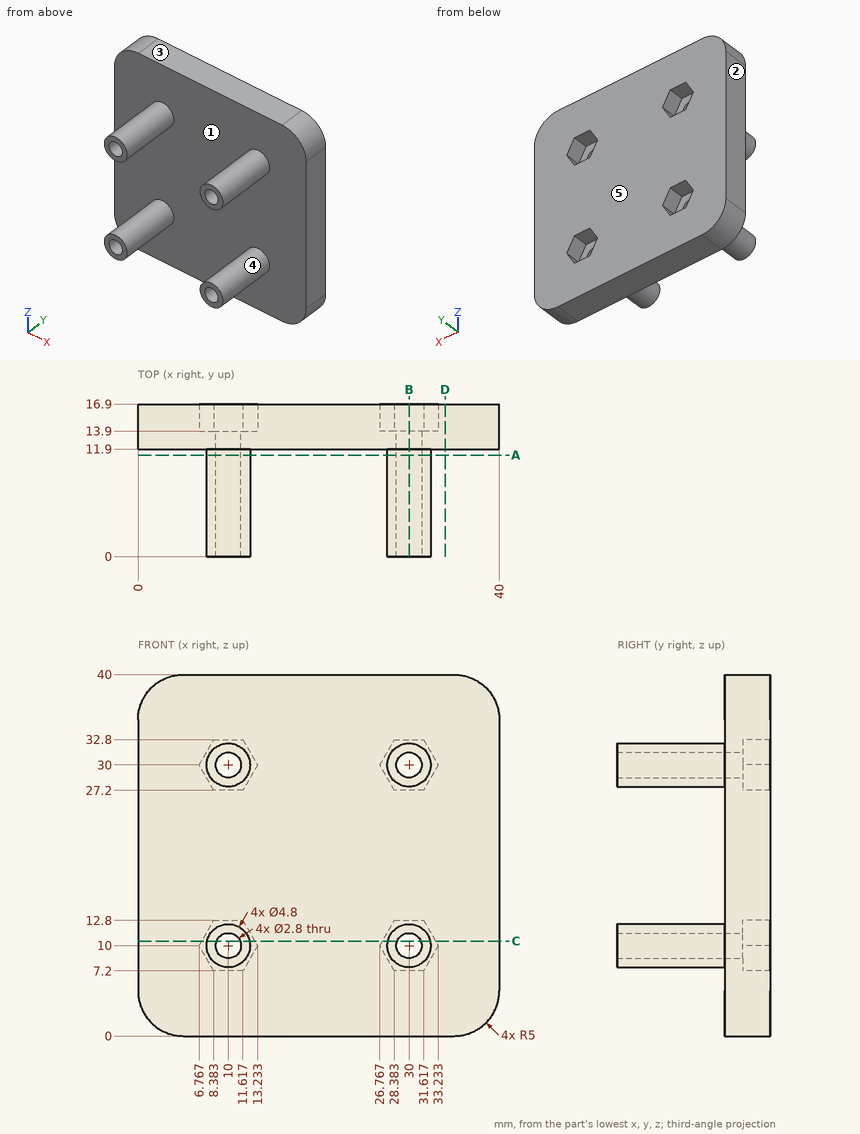
Design review of the part shown in the three views and the two pictorial views. Dimensions are in mm from the part's minimum x, y and z. A direction names the side the tool comes from. Give positions to 0.01 mm unless a question says otherwise; leave off trailing zeros. Order: outer loops, then holes, each group sorted by start corner. A loop starts at its lowest first (then second) coordinate and runs counter-clockwise, first axis right, second up. Notation, with made-up numbers: M -0.5,71 L 9.5,71 A26 cw 9.5,106 Z; hole C 69,1 d1. An arc over 180 degrees is marked long. Answer in a Markdown table with one row per item. Add a question column.
(1) Consider section D-D on x = 34. State the section outline as (y, z) points.
(2) For the marked faces 1 and 2, list the 3-axis set-ups (+Z, -Z, +X, -X, +Y, -Y) from which the entire face can be reached by the end or side of a thin tool; tool diameter is ignored.
(3) Consider section C-C on z = 10.5. State the section outline as (x, y) points (1 decimal).
(4) For pin 1 (3 mm diameter, centred on x = 9.5, z = 11, fed in from +Y); pin 2 (6 mm diameter, centred on y = 5, z = 29, fed in from -X), all flat-tipped, find the tip position at first contact; note any pin that passes through.
(5) Wall thickness on probe 1 along X at (y, z) = (10.5, 10); probe 2 along Z at (x, y) = (31, 12.25): over which ranges is each line inside the solid? List them lowest first. Write a range as [from, to].
(6) Consider section B-B on x = 30. State the section outline as (y, z) points, and give its area (3 significant figures).
(7) Mouldability with a two-part tool opening along Z and no side actions: class the marked faces 3, 4 and 5 as +Z half, -Z half, draft (parallel to the pull), parting line (faces both ways), or undercut.
(8) Consider section A-A on y = 11.25. State the section outline as (x, z) points.
Evaluation:
| question | item | result |
|---|---|---|
| 1 | outline | M 11.9,0 L 16.9,0 L 16.9,40 L 11.9,40 Z |
| 2 | face 1 | -Y |
| 2 | face 2 | +Z, -Z, -X, +Y, -Y |
| 3 | outline | M 0,11.9 L 7.7,11.9 L 7.7,0 L 8.7,0 L 8.7,13.9 L 7.1,13.9 L 7.1,16.9 L 0,16.9 Z; M 11.3,0 L 12.3,0 L 12.3,11.9 L 27.7,11.9 L 27.7,0 L 28.7,0 L 28.7,13.9 L 27.1,13.9 L 27.1,16.9 L 12.9,16.9 L 12.9,13.9 L 11.3,13.9 Z; M 31.3,0 L 32.3,0 L 32.3,11.9 L 40,11.9 L 40,16.9 L 32.9,16.9 L 32.9,13.9 L 31.3,13.9 Z |
| 4 | pin 1 | stops at y = 13.9 |
| 4 | pin 2 | stops at x = 7.6 |
| 5 | probe 1 | x = [7.6, 8.6], [11.4, 12.4], [27.6, 28.6], [31.4, 32.4] |
| 5 | probe 2 | z = [0, 9.02], [10.98, 29.02], [30.98, 40] |
| 6 | outline | M 0,7.6 L 11.9,7.6 L 11.9,0 L 16.9,0 L 16.9,7.2 L 13.9,7.2 L 13.9,8.6 L 0,8.6 Z; M 0,11.4 L 13.9,11.4 L 13.9,12.8 L 16.9,12.8 L 16.9,27.2 L 13.9,27.2 L 13.9,28.6 L 0,28.6 L 0,27.6 L 11.9,27.6 L 11.9,12.4 L 0,12.4 Z; M 0,31.4 L 13.9,31.4 L 13.9,32.8 L 16.9,32.8 L 16.9,40 L 11.9,40 L 11.9,32.4 L 0,32.4 Z |
| 6 | area | 203 mm^2 |
| 7 | face 3 | +Z half |
| 7 | face 4 | undercut |
| 7 | face 5 | draft |
| 8 | outline | C 10,10 d4.8; C 10,30 d4.8; C 30,10 d4.8; C 30,30 d4.8; hole C 10,10 d2.8; hole C 10,30 d2.8; hole C 30,10 d2.8; hole C 30,30 d2.8 |
